from build123d import *

# Parameters (mm, degrees)
BOSS_EXTRUDE1_DEPTH = 25
CUT_EXTRUDE1_DEPTH  = 75
SKETCH3_R           = 25
SKETCH3_R_2         = 12.5
BOSS_EXTRUDE2_DEPTH = 30
RIB2_REACH          = 129.02
SKETCH5_WALL_W      = 284.323638276
SKETCH5_WALL_H      = 6
CIRPATTERN1_COUNT   = 3


with BuildPart() as part:
    # Sketch1 → Boss-Extrude1 (new body)
    with BuildSketch(Plane(origin=(0, 0, 0), x_dir=(1, 0, 0), z_dir=(0, 1, 0))):
        with BuildLine():
            Line((-50, 50), (50, 50))
            ThreePointArc((50, 50), (100, 0), (50, -50))
            Line((50, -50), (-50, -50))
            Line((-50, -50), (-50, 50))
        make_face()
    extrude(amount=BOSS_EXTRUDE1_DEPTH)

    # Sketch2 → Cut-Extrude1 (cut)
    with BuildSketch(Plane.XY.offset(50)):
        with BuildLine():
            Line((-1.010205144, 25), (-50, 25))
            Line((-50, 25), (-50, 5))
            ThreePointArc((-50, 5), (-23.542486889, 10.192593016), (-1.010205144, 25))
        make_face()
    extrude(amount=-CUT_EXTRUDE1_DEPTH, mode=Mode.SUBTRACT)

    # Sketch3 → Boss-Extrude2 (add)
    with BuildSketch(Plane(origin=(0, 25, 0), x_dir=(1, 0, 0), z_dir=(0, 1, 0))):
        with Locations(Location((52.838951486, 0, 0), (0, 0, 90))):
            Circle(SKETCH3_R)
        with Locations(Location((52.838951486, 0, 0), (0, 0, 270))):
            Circle(SKETCH3_R_2, mode=Mode.SUBTRACT)
    extrude(amount=BOSS_EXTRUDE2_DEPTH)

    # Sketch5 wall → Rib2 (add, up to next)
    with BuildSketch(Plane(origin=(53, 35, 35), x_dir=(0, -0.707106781187, 0.707106781187), z_dir=(0, -0.707106781187, -0.707106781187)), mode=Mode.PRIVATE) as rib2_sk1:
        Rectangle(SKETCH5_WALL_W, SKETCH5_WALL_H)
    rib2_tool1 = extrude(rib2_sk1.sketch, amount=RIB2_REACH, mode=Mode.PRIVATE) - part.part
    rib2 = rib2_tool1.solids().sort_by_distance((53, 35, 35))[0]
    add(rib2)

    # CirPattern1: Rib2 ×3 about axis
    cirpattern1_axis = Axis((52.838951486, 0, 0), (0, 1, 0))
    for i in range(1, CIRPATTERN1_COUNT):
        add(rib2.rotate(cirpattern1_axis, i * 360 / CIRPATTERN1_COUNT))


solid = part.part
Here's how the part is built. I have some questions about the finished solid (model axes, mm). A direction names the side the tool comes from. Coordinates: 2 decimals unless noted, no trailing zeros. Loops run counter-clockwise (first coordinate to the right, second up) from the corner with the lowest first, then second, coordinate; pieces in that order, holes last.
1. If we mould it in two halves opening along X, with no side actions, what happens to faces 6 (the flat face through (78.02, 31.38, -18.19)), 7 (the flat face through (22.68, 35.24, -17.28)), 8 (the flat face through (82.881, 35.242, -17.482))? For each: pulls with the +X half, pulls with the -X half, needs draft (parallel to the pull), parting line crosses it, or undercut.
2. Imagine slicing it at D-D, the plane y = 23. Please give me the cut outline in (x, z).
3. For faces 1 (the flat face through (24, 31, -13)), 2 (the flat face through (-31, 17, -25)), 3 (the flat face through (81.043, 31.372, -13.006)), 4 (the flat face through (27.474, 31.372, -17.923)), 5 (the flat face through (26, 25, -1)), which set-ups out of +Z, -Z, +X, -X, +Y, -Y let a thin tool reach every point of the face, with its end or its side?
4. Imagine slicing it at B-B, the plane y = 33. Please give me the cut outline in (x, z).
5. Imagine slicing it at A-A, the plane z = 0. Please give me the cut outline in (x, y).
6. For P1, Ø5, axis at x = 7, z = 12, coming from the -Y side; P2, Ø12, axis at y = 49, z = -1, coming from the +X side; P3, Ø5, axis at y = 31.5, z = -25.5, coming from the +X side; P4, Ø6, axis at y = 35, z = 38, coming from the -X side, each with a flat end and sliding along its axis, tell me the tip position at first contact or that it passes through.
7. I need wall thicknesses on L1, parallel to X at y = 47.75, z = 0; L2, parallel to Y at x = 8, z = 30; L3, parallel to Z at x = -31, y = 18. Which ranges of each line are inside material? Lowest first, please.
8. Imagine slicing it at C-C, the plane x = -6.5. Please give me the cut outline in (y, z), and give its area (3 significant figures).
Taken from the geometry:
1. face 6: undercut
1. face 7: pulls with the -X half
1. face 8: pulls with the +X half
2. outline: (-50, -50) - (50, -50) arc R50 ccw to (50, 50) - (-3.14, 50) - (-3.14, -25) - (-50, -25) - close
3. face 1: -X, +Y
3. face 2: +Z, -X, +Y
3. face 3: +X, +Y
3. face 4: -Z, +Y
3. face 5: +Y
4. outline: (19.22, -15.76) - (22.22, -20.96) - (32.75, -14.88) arc R25 ccw to (72.74, -15.14) - (83.3, -21.24) - (86.3, -16.04) - (75.77, -9.96) arc R25 ccw to (56, 24.8) - (56, 37) - (50, 37) - (50, 24.84) arc R25 ccw to (29.78, -9.66) - close; hole circle Ø25 at (52.84, 0)
5. outline: (-50, 0) - (100, 0) - (100, 25) - (77.84, 25) - (77.84, 55) - (65.34, 55) - (65.34, 25) - (40.34, 25) - (40.34, 55) - (27.84, 55) - (27.84, 25) - (-1.01, 25) arc R70 cw to (-50, 5) - close
6. P1: stops at y = 0
6. P2: stops at x = 77.84
6. P3: stops at x = 62.64
6. P4: stops at x = 50
7. L1: x = 27.84 to 40.34, 65.34 to 77.84
7. L2: y = 0 to 25
7. L3: z = -50 to -25
8. outline: (0, -50) - (25, -50) - (25, -25) - (20.16, -25) - (20.16, 50) - (0, 50) - close
8. area: 2,140 mm2
